For this review, take the finished solid that the model builds, in its own axes (mm). Coordinates: 2 decimals unless noted, no trailing zeros. Write each loop counter-clockwise with the first axis right and the second up, starting at its lowest first coordinate (ties: lowest second). Pieces come first, ordered by that corner, then holes.
```python
from build123d import *

# Parameters (mm, degrees)
F1_DEPTH = 1.27
F2_R     = 0.635
F4_R     = 1.8415
F5_DEPTH = 1.524
F7_D     = 3.81
F8_R     = 0.3175


with BuildPart() as f1:
    # F0 (on Front) → F1 (new body)
    with BuildSketch(Plane.XZ):
        with BuildLine():
            ThreePointArc((3.175, 3.175), (0.929936, 2.245064), (0, 0))
            ThreePointArc((0, 0), (0.929936, -2.245064), (3.175, -3.175))
            ThreePointArc((3.175, -3.175), (5.420064, -2.245064), (6.35, 0))
            ThreePointArc((6.35, 0), (5.420064, 2.245064), (3.175, 3.175))
        make_face()
        with BuildLine():
            ThreePointArc((3.175, -3.175), (0.929936, -2.245064), (0, 0))
            ThreePointArc((0, 0), (-0.929936, -2.245064), (-3.175, -3.175))
            Line((-3.175, -3.175), (3.175, -3.175))
        make_face()
        with BuildLine():
            ThreePointArc((-3.175, -3.175), (-0.929936, -2.245064), (0, 0))
            ThreePointArc((0, 0), (-0.929936, 2.245064), (-3.175, 3.175))
            ThreePointArc((-3.175, 3.175), (-6.35, 0), (-3.175, -3.175))
        make_face()
        with BuildLine():
            ThreePointArc((-3.175, 3.175), (-0.929936, 2.245064), (0, 0))
            ThreePointArc((0, 0), (0.929936, 2.245064), (3.175, 3.175))
            Line((3.175, 3.175), (-3.175, 3.175))
        make_face()
    extrude(amount=F1_DEPTH)

    # F2
    f2_edges = [f1.edges().sort_by_distance(p)[0] for p in [
        (0, -1.27, 3.175),
        (-6.35, -1.27, 0),
        (6.35, -1.27, 0),
        (0, -1.27, -3.175),
    ]]
    fillet(f2_edges, radius=F2_R)

    # F4 (on face) → F5 (join)
    with BuildSketch(Plane.XZ.offset(1.27)):
        with Locations((3.175, 0)):
            Circle(F4_R)
    extrude(amount=F5_DEPTH)

    # F7 (through all)
    with Locations(Plane.XZ.offset(1.27)):
        with Locations((-3.175, 0)):
            Hole(F7_D / 2)

    # F8
    f8_edges = [f1.edges().sort_by_distance(p)[0] for p in [
        (1.3335, -2.794, 0),
    ]]
    fillet(f8_edges, radius=F8_R)


solid = f1.part
```
Q1. Clearance check with flat-ended pins moving along their axes: pin 1 Ø1.5 at (y, z) = (-2.5, 0.5) entering from +X; pin 2 Ø2.5 at (x, z) = (-3.175, 0) entering from +Y; pin 3 Ø1 at (x, y) = (4.5, -0.5) entering from +Z. State where each tip first meets the part, or that it passes through.
Ans:
pin 1: stops at x = 5.02
pin 2: passes through
pin 3: stops at z = 3.07
Q2. Draft analysis for pull direction Z (two halves, no side actions). For faces 1 (the cylindrical face through (4.025, -1.865, -1.634)), 2 (the cylindrical face through (-1.663, -0.626, -1.159)), 3 (the flat face through (1, 0, 0)), state which applies: +Z half, -Z half, draft (parallel to the pull), parting line (faces both ways), or undercut.
Ans:
face 1: parting line
face 2: undercut
face 3: draft
Q3. For probe 1 along Y at (x, z) = (1.25, 1.5); probe 2 along Z at (x, y) = (-1.5, -0.6) (3 decimals); probe 3 along Z at (x, y) = (0.25, -0.7), list the stretches that pass through material, from the lowest coordinate up.
Ans:
probe 1: y = -1.27 to 0
probe 2: z = -3.175 to -0.907, 0.907 to 3.175
probe 3: z = -3.17 to 3.17
Q4. Add section A-A (y = -0.3). State the section outline as (x, z) points (3 decimals).
Ans:
outline: (-3.175, -3.175) - (3.175, -3.175) arc R3.175 ccw to (3.175, 3.175) - (-3.175, 3.175) arc R3.175 ccw to start; hole circle Ø3.81 at (-3.175, 0)
Q5. Add section C-C (y = -2.2). State the section outline as (x, z) points (1 decimal).
Ans:
outline: circle Ø3.7 at (3.2, 0)
Q6. Add section D-D (y = -0.95). State the section outline as (x, z) points (3 decimals), then the cut area to 3 significant figures.
Ans:
outline: (-3.175, -3.091) - (3.175, -3.091) arc R3.091 ccw to (3.175, 3.091) - (-3.175, 3.091) arc R3.091 ccw to start; hole circle Ø3.81 at (-3.175, 0)
area: 57.9 mm2
Q7. Add section B-B (x = -1). State the section outline as (y, z) points (3 decimals), then the cut area to 3 significant figures.
Ans:
outline: (-1.27, -2.54) arc R0.635 ccw to (-0.635, -3.175) - (0, -3.175) - (0, 3.175) - (-0.635, 3.175) arc R0.635 ccw to (-1.27, 2.54) - close
area: 7.89 mm2
